Design review of the part built by this model. Coordinates are the model's own, in mm. Face numbers are marked on the shaded views. A direction names the side the tool comes from. Round coordinates to 2 decimals unless told otherwise and drop trailing zeros. Loops run counter-clockwise (first coordinate to the right, second up) from the corner with the lowest first, then second, coordinate; pieces in that order, holes last. Notation, with made-up numbers: M 53.5,58 L 112.5,58 A27 ccw 112.5,90 Z; hole C 13.5,23.25 d6. An arc over 180 degrees is marked long. Answer as CSV lines item,"result". Start each with the question number.
from build123d import *

# Parameters (mm, degrees)
SKETCH1_W               = 15.875
SKETCH1_H               = 25.4
BOSS_EXTRUDE1_DEPTH     = 4.318
BOSS_EXTRUDE2_START     = 4.318
SKETCH1_3_W             = 15.875
SKETCH1_3_H             = 25.4
BOSS_EXTRUDE2_DEPTH     = 10.16
CUT_EXTRUDE1_DEPTH      = 66.211748481
CUT_EXTRUDE1_DEPTH_BACK = 66.211748481
SKETCH2_W               = 6.35
SKETCH2_H               = 6.35


with BuildPart() as part:
    # Sketch1 → Boss-Extrude1 (new body)
    # profile 1 of 2: a face of its own
    with BuildSketch(Plane(origin=(0, 0, 0), x_dir=(1, 0, 0), z_dir=(0, 1, 0))):
        Polygon((44.45, 0), (0, 0), (0, -45.466), (14.2875, -45.466), (14.2875, -20.066), (30.1625, -20.066), (30.1625, -45.466), (44.45, -45.466), align=None)
        with BuildLine():
            ThreePointArc((4.8895, -29.591), (6.4135, -28.067), (7.9375, -29.591))
            Line((7.9375, -29.591), (7.9375, -41.148))
            ThreePointArc((7.9375, -41.148), (6.4135, -42.672), (4.8895, -41.148))
            Line((4.8895, -41.148), (4.8895, -29.591))
        make_face(mode=Mode.SUBTRACT)
        with BuildLine():
            ThreePointArc((36.5125, -29.591), (38.0365, -28.067), (39.5605, -29.591))
            Line((39.5605, -29.591), (39.5605, -41.148))
            ThreePointArc((39.5605, -41.148), (38.0365, -42.672), (36.5125, -41.148))
            Line((36.5125, -41.148), (36.5125, -29.591))
        make_face(mode=Mode.SUBTRACT)
        with BuildLine():
            ThreePointArc((4.8895, -4.064), (6.4135, -2.54), (7.9375, -4.064))
            Line((7.9375, -4.064), (7.9375, -15.621))
            ThreePointArc((7.9375, -15.621), (6.4135, -17.145), (4.8895, -15.621))
            Line((4.8895, -15.621), (4.8895, -4.064))
        make_face(mode=Mode.SUBTRACT)
        with BuildLine():
            ThreePointArc((36.5125, -4.064), (38.0365, -2.54), (39.5605, -4.064))
            Line((39.5605, -4.064), (39.5605, -15.621))
            ThreePointArc((39.5605, -15.621), (38.0365, -17.145), (36.5125, -15.621))
            Line((36.5125, -15.621), (36.5125, -4.064))
        make_face(mode=Mode.SUBTRACT)
    # profile 2 of 2: a face of its own
    with BuildSketch(Plane(origin=(0, 0, 0), x_dir=(1, 0, 0), z_dir=(0, 1, 0))):
        with Locations((22.225, -32.766)):
            Rectangle(SKETCH1_W, SKETCH1_H)
    extrude(amount=BOSS_EXTRUDE1_DEPTH)

    # Sketch1<3> → Boss-Extrude2 (add)
    with BuildSketch(Plane(origin=(0, 0, 0), x_dir=(1, 0, 0), z_dir=(0, 1, 0)).offset(BOSS_EXTRUDE2_START)):
        with Locations((22.225, -32.766)):
            Rectangle(SKETCH1_3_W, SKETCH1_3_H)
    extrude(amount=BOSS_EXTRUDE2_DEPTH)

    # Sketch2 → Cut-Extrude1 (cut, two sides: drawn at the far end of the back side and taken through both)
    with BuildSketch(Plane.XY.offset(45.466).offset(-CUT_EXTRUDE1_DEPTH_BACK)):
        with Locations((22.225, 11.303)):
            Rectangle(SKETCH2_W, SKETCH2_H)
    extrude(amount=CUT_EXTRUDE1_DEPTH + CUT_EXTRUDE1_DEPTH_BACK, mode=Mode.SUBTRACT)


solid = part.part
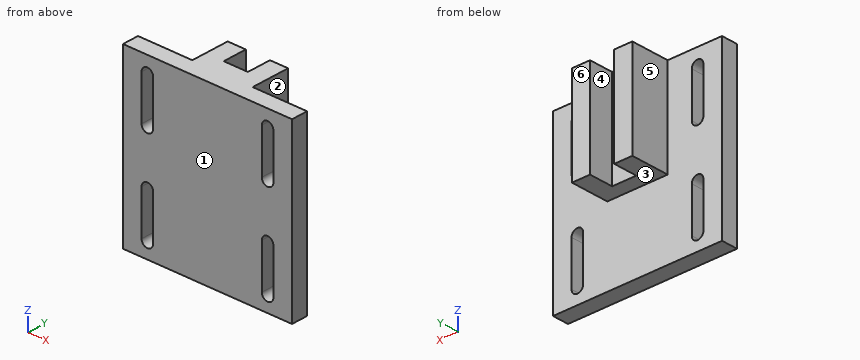
Item 1: Consider section B-B, the plane y = 10. Write out the cut boundary in (x, z).
Item 2: Insertion check: pin 1 Ø4.5 at (y, z) = (2, 35.5) entering from -X; pin 2 Ø1.9 at (y, z) = (11.5, 28.5) entering from +X; pin 3 Ø1 at (x, z) = (26.5, 9.5) entering from +Y; pin 4 Ø5 at (y, z) = (11.5, 36) entering from -X. Each pin has a flat end and moves straight along its axis. Give the tip position at first contact, or say it passes through.
Item 3: Tool access review of the marked faces 1, 2 and 3: name each direction out of +Z, -Z, +X, -X, +Y, -Y from which nothing blocks a thin tool from reaching the whole face with its end or side.
Item 4: The part is to be moulded in two halves that separate along X. For the marked faces 4, 5 and 6, say which applies: +X half, -X half, draft (parallel to the pull), parting line (faces both ways), or undercut.
Item 5: Consider section C-C, the plane y = 1.25. Write out the cut boundary in (x, z), then the cut area to 3 significant figures.
Item 6: To check wall thickness, follow line 1 (X direction, y = 3, z = 8); line 2 (X direction, y = 12.5, z = 31.5); line 3 (Y direction, x = 37.5, z = 28). State the ranges of each line that lie inside material, in increasing order.
Item 7: Consider section A-A, the plane z = 10. Write out the cut boundary in (x, y), then the cut area to 3 significant figures.
Item 8: Consider section D-D, the plane z = 26.5. Write out the cut boundary in (x, y).
Found:
1,outline,"M 14.29,20.07 L 19.05,20.07 L 19.05,45.47 L 14.29,45.47 Z; M 25.4,20.07 L 30.16,20.07 L 30.16,45.47 L 25.4,45.47 Z"
2,pin 1,"stops at x = 0"
2,pin 2,"stops at x = 30.16"
2,pin 3,"stops at y = 4.32"
2,pin 4,"stops at x = 14.29"
3,face 1,"+Z, -Z, +X, -X, -Y"
3,face 2,"+Z, -Z, +X, +Y"
3,face 3,"-Z, +X, -X, +Y"
4,face 4,"undercut"
4,face 5,"-X half"
4,face 6,"draft"
5,outline,"M 0,0 L 44.45,0 L 44.45,45.47 L 0,45.47 Z; hole M 4.89,4.06 A1.52 ccw 7.94,4.06 L 7.94,15.62 A1.52 ccw 4.89,15.62 Z; hole M 4.89,29.59 A1.52 ccw 7.94,29.59 L 7.94,41.15 A1.52 ccw 4.89,41.15 Z; hole M 36.51,4.06 A1.52 ccw 39.56,4.06 L 39.56,15.62 A1.52 ccw 36.51,15.62 Z; hole M 36.51,29.59 A1.52 ccw 39.56,29.59 L 39.56,41.15 A1.52 ccw 36.51,41.15 Z"
5,area,"1,850 mm^2"
6,line 1,"x = 0 to 4.89, 7.94 to 36.51, 39.56 to 44.45"
6,line 2,"x = 14.29 to 19.05, 25.4 to 30.16"
6,line 3,"y = 0 to 4.32"
7,outline,"M 0,0 L 4.89,0 L 4.89,4.32 L 0,4.32 Z; M 7.94,0 L 36.51,0 L 36.51,4.32 L 7.94,4.32 Z; M 39.56,0 L 44.45,0 L 44.45,4.32 L 39.56,4.32 Z"
7,area,"166 mm^2"
8,outline,"M 0,0 L 44.45,0 L 44.45,4.32 L 30.16,4.32 L 30.16,14.48 L 25.4,14.48 L 25.4,8.13 L 19.05,8.13 L 19.05,14.48 L 14.29,14.48 L 14.29,4.32 L 0,4.32 Z"
